The drawing under review shows one solid part. Ordinate dimensions are in mm from its lowest x, y, z. A direction names the side the tool comes from. Give positions to 0.01 mm unless a question says otherwise; leave off trailing zeros. Write each loop counter-clockwise with the first axis right and the second up, starting at its lowest first coordinate (ties: lowest second). Pieces come first, ordered by that corner, then holes. Notation, with made-up numbers: (59.5, 52) -> (64.5, 52) arc R16 cw to (64.5, 72) -> close; hole circle Ø11 at (10.25, 61). An arc over 180 degrees is marked (long way). Put each result on its own line as item: value. Start each with the question number.
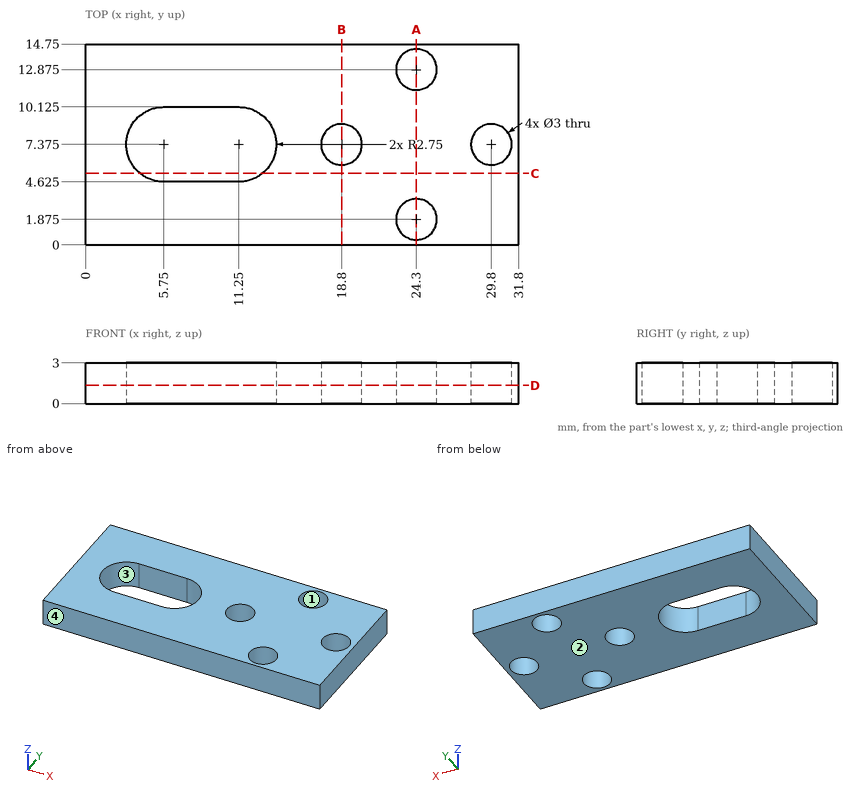
Q1. Mouldability with a two-part tool opening along X and no side actions: class the marked faces 1 and 2 as +X half, -X half, draft (parallel to the pull), parting line (faces both ways), or undercut.
Q2. Take a section at A-A on x = 24.3. Give the boundary of the cut face in (y, z) (3 decimals).
Q3. Take a section at D-D on z = 1.35. Give the boundary of the cut face in (x, y) (3 decimals).
Q4. To check wall thickness, follow probe 1 along Y at (x, z) = (9.5, 0.95) (3 decimals); probe 2 along Y at (x, z) = (18.8, 2.3) (3 decimals); probe 3 along X at (y, z) = (2, 1.8). State the ranges of each line that lie inside material, in increasing order. Write a range as from..to.
Q5. Machinability: for the marked faces 3 and 4, which of the approach directions +Z, -Z, +X, -X, +Y, -Y give a long, thin tool a straight path to every point of the face, cutting with its end or side? Answer none if there is none.
Q6. Take a section at B-B on x = 18.8. Give the boundary of the cut face in (y, z) (3 decimals), then the cut area to 4 significant figures.
Q7. Take a section at C-C on y = 5.25. Give the boundary of the cut face in (x, z).
Result:
1. face 1: undercut
1. face 2: draft
2. outline: (0, 0) -> (0.375, 0) -> (0.375, 3) -> (0, 3) -> close; (3.375, 0) -> (11.375, 0) -> (11.375, 3) -> (3.375, 3) -> close; (14.375, 0) -> (14.75, 0) -> (14.75, 3) -> (14.375, 3) -> close
3. outline: (0, 0) -> (31.8, 0) -> (31.8, 14.75) -> (0, 14.75) -> close; hole (5.75, 4.625) -> (11.25, 4.625) arc R2.75 ccw to (11.25, 10.125) -> (5.75, 10.125) arc R2.75 ccw to start; hole circle Ø3 at (18.8, 7.375); hole circle Ø3 at (24.3, 1.875); hole circle Ø3 at (24.3, 12.875); hole circle Ø3 at (29.8, 7.375)
4. probe 1: y = 0..4.625, 10.125..14.75
4. probe 2: y = 0..5.875, 8.875..14.75
4. probe 3: x = 0..22.81, 25.79..31.8
5. face 3: +Z, -Z
5. face 4: +Z, -Z, +X, -X, -Y
6. outline: (0, 0) -> (5.875, 0) -> (5.875, 3) -> (0, 3) -> close; (8.875, 0) -> (14.75, 0) -> (14.75, 3) -> (8.875, 3) -> close
6. area: 35.25 mm^2
7. outline: (0, 0) -> (4, 0) -> (4, 3) -> (0, 3) -> close; (13, 0) -> (31.8, 0) -> (31.8, 3) -> (13, 3) -> close
